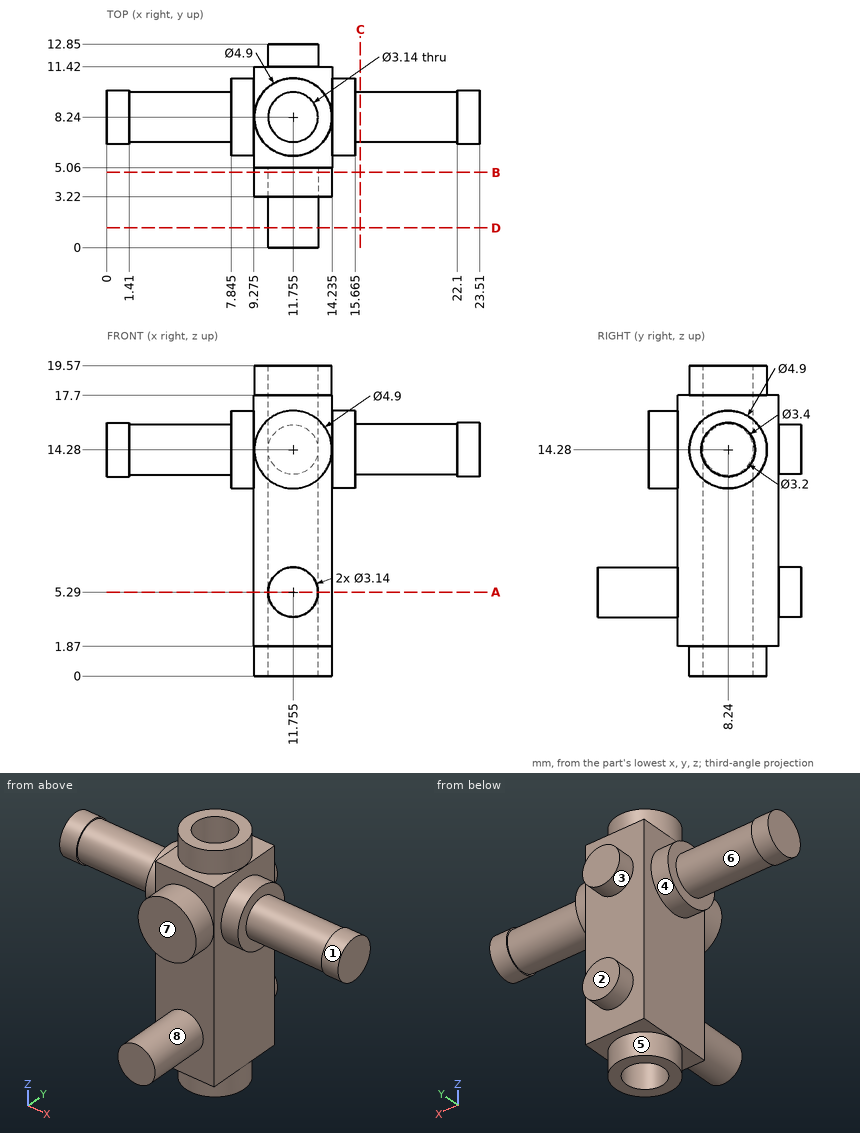
Check sheet for the drawn part. Datum: minimum x, y, z corner. Units: mm. A direction names the side the tool comes from. Round coordinates to 2 decimals unless told otherwise and drop trailing zeros. Loops run counter-clockwise (first coordinate to the right, second up) from the corner with the lowest first, then second, coordinate; pieces in that order, holes last. Notation, with made-up numbers: (-13, 69) - (44, 69) arc R19 ccw to (44, 92) - close; hole circle Ø4 at (7.25, 20). An arc over 180 degrees is marked (long way). Answer as a JSON object with one key per item and string values. Group by question number.
Q1. Gauge pin test, flat ends, axial feed: P1, Ø3, axis at x = 17.5, y = 6.5, coming from the -Z side; P2, Ø4, axis at y = 7, z = 15, coming from the -X side; P3, Ø4, axis at x = 3, y = 5, coming from the +Z side; P4, Ø7, axis at y = 7.5, z = 9, coming from the -X side (3 decimals). Record the tip position at first contact, or that the pin passes through.
Q2. Scan lines: line 1 along X through (y, z) = (8.24, 13.5) (3 decimals); line 2 along X through (y, z) = (8.24, 4.5) (3 decimals); line 3 along Y through (x, z) = (11.75, 8.75). Record each from-to range of solid material in increasing order. Write a range as [from, to].
Q3. Sectioned sample at A-A, the plane z = 5.29. Enter the section's corners in (x, y) (3 decimals).
Q4. Sectioned sample at C-C, the plane x = 16. Enter the section's corners in (y, z), plus the area to 3 significant figures.
Q5. Mould release check, pull along Z, two halves, no side actions. Record for the marked faces 1, 2 and 3: released by +Z, released by -Z, zero draft, split by the parting line, or undercut.
Q6. Sectioned sample at B-B, the plane y = 4.75. Enter the section's corners in (x, z) (3 decimals), plus the area to 3 significant figures.
Q7. Set-up check for the marked faces 4, 5, 6, 7 and 8: record each of +Z, -Z, +X, -X, +Y, -Y from which the full face is reachable in a straight line by a thin tool's end or side.
Q8. Sectioned sample at D-D, the plane y = 1.25. Enter the section's corners in (x, z) (3 decimals).
Solution:
{
 "1": {"P1": "stops at z = 12.7", "P2": "stops at x = 0", "P3": "stops at z = 15.29", "P4": "stops at x = 7.845"},
 "2": {"line 1": "x = [0, 10.185], [13.325, 23.51]", "line 2": "x = [9.275, 10.185], [13.325, 14.235]", "line 3": "y = [5.06, 6.67], [9.81, 11.42]"},
 "3": {"outline": "(9.275, 5.06) - (10.185, 5.06) - (10.185, 0) - (13.325, 0) - (13.325, 5.06) - (14.235, 5.06) - (14.235, 11.42) - (13.325, 11.42) - (13.325, 12.85) - (10.185, 12.85) - (10.185, 11.42) - (9.275, 11.42) - close; hole circle Ø3.14 at (11.755, 8.24)"},
 "4": {"outline": "circle Ø3.2 at (8.24, 14.28)", "area": "8.04 mm²"},
 "5": {"face 1": "split by the parting line", "face 2": "zero draft", "face 3": "undercut"},
 "6": {"outline": "circle Ø4.9 at (11.755, 14.28); circle Ø3.14 at (11.755, 5.29)", "area": "26.6 mm²"},
 "7": {"face 4": "-X", "face 5": "-Z", "face 6": "none", "face 7": "+Z, +X, -X, -Y", "face 8": "-Y"},
 "8": {"outline": "circle Ø3.14 at (11.755, 5.29)"}
}
